Here's how the part is built. I have some questions about the finished solid (model axes, mm). A direction names the side the tool comes from. Round coordinates to 2 decimals unless told otherwise and drop trailing zeros. Loops run counter-clockwise (first coordinate to the right, second up) from the corner with the lowest first, then second, coordinate; pieces in that order, holes last. Notation, with made-up numbers: M -15,39.5 L 44,39.5 A27 cw 44,63.5 Z; hole C 46.5,82 d4. An arc over 180 degrees is marked long. Put each result on its own line as item: value. Start each with the question number.
```python
from build123d import *

# Parameters (mm, degrees)
SKETCH1_R           = 50
BOSS_EXTRUDE1_DEPTH = 60
SKETCH2_R           = 15
BOSS_EXTRUDE2_DEPTH = 12.5
DOME1_FACE_RADIUS   = 50
DOME1_HEIGHT        = 50


with BuildPart() as part:
    # Sketch1 → Boss-Extrude1 (new body)
    with BuildSketch(Plane(origin=(0, 0, 0), x_dir=(1, 0, 0), z_dir=(0, 1, 0))):
        with Locations(Location((0, 0, 0), (0, 0, 270))):
            Circle(SKETCH1_R)
    extrude(amount=BOSS_EXTRUDE1_DEPTH)

    # Sketch2 → Boss-Extrude2 (add, symmetric)
    with BuildSketch(Plane(origin=(0, 0, 0), x_dir=(0, 0, -1), z_dir=(1, 0, 0))):
        with BuildLine():
            Line((-25, 100), (-25, 60))
            Line((-25, 60), (25, 60))
            Line((25, 60), (25, 100))
            ThreePointArc((25, 100), (0, 125), (-25, 100))
        make_face()
        with Locations((0, 100)):
            Circle(SKETCH2_R, mode=Mode.SUBTRACT)
    extrude(amount=BOSS_EXTRUDE2_DEPTH, both=True)

    # Dome1: a dome of height H over a round flat face of radius A is a cap of a sphere of radius (A * A + H * H) / (2 * H)
    dome1_r = (DOME1_FACE_RADIUS * DOME1_FACE_RADIUS + DOME1_HEIGHT * DOME1_HEIGHT) / (2 * DOME1_HEIGHT)
    dome1_base = Plane((0, 0, 0), z_dir=(0, -1, 0))
    with Locations(dome1_base.offset(DOME1_HEIGHT - dome1_r)):
        dome1_ball = Sphere(dome1_r, mode=Mode.PRIVATE)
    add(split(dome1_ball, bisect_by=dome1_base, keep=Keep.TOP, mode=Mode.PRIVATE))


solid = part.part
```
1) I'm going to push flat-ended pins straight in: P1, Ø3, axis at y = 53, z = 10, coming from the -X side; P2, Ø3, axis at x = -8.5, y = 44, coming from the -Z side; P3, Ø6, axis at y = 31.5, z = -2.5, coming from the -X side. Where does each tip first touch, or does it pass through?
2) On a 3-axis mill with a long thin cutter (end or side, diameter ignored), from which of +Z, -Z, +X, -X, +Y, -Y can I reach the whole of each face in a straight line? I mean faces 4 (the face through (0, 80, 25)), 5 (the face through (12.5, 86, 6)), 6 (the face through (-12.5, 86, 6)). Say none if no direction works.
3) Suppose I cut it at D-D (x = -10.5). Write out the boundary of the cut face in (y, z).
4) Suppose I cut it at B-B (x = 0). Write out the boundary of the cut face in (y, z).
5) Suppose I cut it at C-C (y = 32). Write out the boundary of the cut face in (x, z), plus the area to 3 significant figures.
6) If we mould it in two halves opening along Y, with no side actions, what happens to faces 1 (the face through (-0.175, 85.357, 3.252)), 2 (the face through (0.175, 124.994, -0.55)), 3 (the face through (0, 80, -25))? For each: pulls with the +Y half, pulls with the -Y half, needs draft (parallel to the pull), parting line crosses it, or undercut.
7) If I drill on probe 1 along Y at (x, z) = (3.25, 0); probe 2 along X at (y, z) = (67, -9.5); probe 3 along Y at (x, z) = (6, 0), over which ranges is the centre line in solid material (lowest first)? Write a range as from..to.
8) Suppose I cut it at A-A (z = 0). Write out the boundary of the cut face in (x, y).
Results are:
1. P1: x = -49.27
1. P2: z = -49.51
1. P3: x = -50
2. face 4: +Z, +X, -X, +Y
2. face 5: +Z, -Z, +X, +Y
2. face 6: +Z, -Z, -X, +Y
3. outline: M 0,-48.89 L 60,-48.89 L 60,-25 L 100,-25 A25 ccw 100,25 L 60,25 L 60,48.89 L 0,48.89 A48.89 ccw Z; hole C 100,0 d30
4. outline: M 0,-50 L 60,-50 L 60,-25 L 100,-25 A25 ccw 100,25 L 60,25 L 60,50 L 0,50 A50 ccw Z; hole C 100,0 d30
5. outline: C 0,0 d100
5. area: 7,850 mm²
6. face 1: undercut
6. face 2: pulls with the +Y half
6. face 3: needs draft
7. probe 1: -49.89..85, 115..125
7. probe 2: -12.5..12.5
7. probe 3: -49.64..85, 115..125
8. outline: M -50,0 A50 ccw 50,0 L 50,60 L 12.5,60 L 12.5,85 L -12.5,85 L -12.5,60 L -50,60 Z; M -12.5,115 L 12.5,115 L 12.5,125 L -12.5,125 Z
